Study the drawing (mm; zero at the part's minimum x, y, z) and answer. A direction names the side the tool comes from. Give positions to 0.01 mm unless a question says otherwise; leave off trailing zeros. Write each loop counter-clockwise with the first axis right and the second up, starting at its lowest first coordinate (ties: lowest second). Pieces come first, ordered by that corner, then holes. Notation, with made-up numbers: (54.25, 4) - (106.25, 4) arc R14 cw to (106.25, 11) - close; hole circle Ø4 at (74, -28). An arc over 180 degrees is marked (long way). Answer in a Markdown table with one row per item. Add a question column.
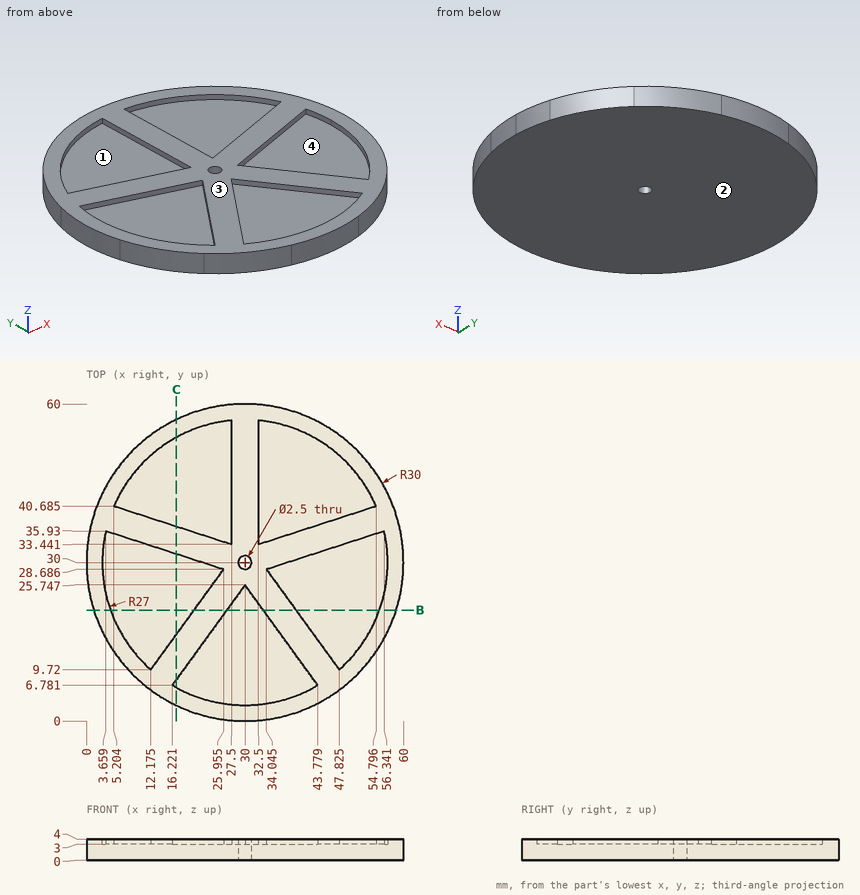
1. Section B-B (y = 21) is taken. Give the vertices of the cut face in (x, z) (1 decimal).
2. Straight lines are drawn through the part: L1, parallel to Y at x = 30, z = 2.55; L2, parallel to Z at x = 36, y = 53; L3, parallel to X at y = 7, z = 3.75. For each, find the intervals that lie inside material, in ascending order. Write a range as [from, to].
3. The mould has two halves that part along X. Classify the marked faces 1 and 2: +X half, -X half, draft (parallel to the pull), parting line (faces both ways), or undercut.
4. Section C-C (x = 17) is taken. Give the vertices of the cut face in (y, z) (1 decimal).
5. Given pin 1 Ø7 at (x, y) = (14, 27) entering from +Z; pin 2 Ø1 at (y, z) = (34.5, 1) entering from -X; pin 3 Ø2 at (y, z) = (9, 2.5) entering from +X, each flat-ended and moving along its own axis, determine where each tip first touches the part or whether it passes through.
6. A tool of negligible diameter and unlimited length cuts with its end or side. For the marked faces 3 and 4, from which of +Z, -Z, +X, -X, +Y, -Y can it reach the whole face along a straight path? Write none if from no direction.
Geometry check:
| question | item | result |
|---|---|---|
| 1 | outline | (1.4, 0) - (58.6, 0) - (58.6, 4) - (55.5, 4) - (55.5, 3) - (39.6, 3) - (39.6, 4) - (33.4, 4) - (33.4, 3) - (26.6, 3) - (26.6, 4) - (20.4, 4) - (20.4, 3) - (4.5, 3) - (4.5, 4) - (1.4, 4) - close |
| 2 | L1 | [0, 28.75], [31.25, 60] |
| 2 | L2 | [0, 3] |
| 2 | L3 | [10.74, 16.38], [43.62, 49.26] |
| 3 | face 1 | undercut |
| 3 | face 2 | draft |
| 4 | outline | (3, 0) - (57, 0) - (57, 4) - (53.7, 4) - (53.7, 3) - (36.9, 3) - (36.9, 4) - (31.6, 4) - (31.6, 3) - (16.4, 3) - (16.4, 4) - (7.9, 4) - (7.9, 3) - (6.3, 3) - (6.3, 4) - (3, 4) - close |
| 5 | pin 1 | z = 3 |
| 5 | pin 2 | x = 0.27 |
| 5 | pin 3 | x = 52.36 |
| 6 | face 3 | +Z, +X, -X, +Y, -Y |
| 6 | face 4 | +Z |
